from build123d import *

# Parameters (mm, degrees)
F1_DEPTH  = 1
F0_W      = 50
F0_H      = 23.8363201171
F0_W_2    = 35
F2_DEPTH  = 4
F3_W      = 50
F3_H      = 5
F3_H_2    = 13.8363201171
F4_DEPTH  = 20
F6_DEPTH  = 50
F7_W      = 4
F7_H      = 10
F7_H_2    = 6.0470494551
F8_DEPTH  = 12
F9_START  = -7
F7_W_2    = 1.75
F9_DEPTH  = 5
F10_W     = 23
F10_H     = 5
F11_DEPTH = 45


with BuildPart() as f1:
    # F0 (on Top) → F1 (new body)
    with BuildSketch(Plane.XY):
        Polygon((-50, 46.1636798829), (-50, 23.8363201171), (-25, 23.8363201171), (25, 23.8363201171), (50, 23.8363201171), (50, 46.1636798829), (15, 46.1636798829), (15, 70), (-15, 70), (-15, 46.1636798829), align=None)
    extrude(amount=F1_DEPTH)

    # F0 (on Top) → F2 (join)
    with BuildSketch(Plane.XY):
        with Locations((0, 11.9181600586)):
            Rectangle(F0_W, F0_H)
        with Locations((32.5, 58.0818399414)):
            Rectangle(F0_W_2, F0_H)
        with Locations((-32.5, 58.0818399414)):
            Rectangle(F0_W_2, F0_H)
    extrude(amount=F2_DEPTH)

    # F3 (on face) → F4 (join)
    with BuildSketch(Plane.XY.offset(4)):
        with Locations((0, 21.3363201171)):
            Rectangle(F3_W, F3_H)
        with Locations((0, 11.9181600586)):
            Rectangle(F3_W, F3_H_2)
        with Locations((0, 2.5)):
            Rectangle(F3_W, F3_H)
    extrude(amount=F4_DEPTH)

    # F5 (on face) → F6 (cut)
    with BuildSketch(Plane.YZ.offset(25)):
        Polygon((0, 24), (0, 4), (5, 24), align=None)
        Polygon((22.7283012867, 19.5679246783), (18.8363201171, 4), (23.8363201171, 4), (23.8363201171, 24), align=None)
        Polygon((23.8363201171, 24), (5, 24), (22.7283012867, 19.5679246783), align=None)
    extrude(amount=-F6_DEPTH, mode=Mode.SUBTRACT)

    # F7 (on face) → F8 (cut)
    with BuildSketch(Plane(origin=(0, 16.7871248161, -4.196781204), x_dir=(-1, 0, 0), z_dir=(0, 0.9701425001, -0.242535625))):
        with Locations((0, 19.4960981287)):
            Rectangle(F7_W, F7_H)
        with Locations((0, 11.4725734011)):
            Rectangle(F7_W, F7_H_2)
    extrude(amount=-F8_DEPTH, mode=Mode.SUBTRACT)

    # F7 (on face) → F9 (cut)
    with BuildSketch(Plane(origin=(0, 16.7871248161, -4.196781204), x_dir=(-1, 0, 0), z_dir=(0, 0.9701425001, -0.242535625)).offset(F9_START)):
        with Locations((2.875, 19.4960981287)):
            Rectangle(F7_W_2, F7_H)
        with Locations((-2.875, 19.4960981287)):
            Rectangle(F7_W_2, F7_H)
    extrude(amount=-F9_DEPTH, mode=Mode.SUBTRACT)

    # F10 (on face) → F11 (join)
    with BuildSketch(Plane(origin=(0, 5.9411764706, 23.7647058824), x_dir=(1, 0, 0), z_dir=(0, 0.242535625, 0.9701425001))):
        Polygon((40, 17.3037721918), (25, 17.3037721918), (25, 12.3037721918), (35, 12.3037721918), (35, -7.6962278082), (40, -7.6962278082), align=None)
        with Locations((13.5, 14.8037721918)):
            Rectangle(F10_W, F10_H)
        with Locations((-13.5, 14.8037721918)):
            Rectangle(F10_W, F10_H)
        Polygon((-25, 17.3037721918), (-40, 17.3037721918), (-40, -7.6962278082), (-35, -7.6962278082), (-35, 12.3037721918), (-25, 12.3037721918), align=None)
    extrude(amount=F11_DEPTH)


solid = f1.part
Could you check a few things on this model? Use its own coordinates, in mm. A direction names the side the tool comes from. Give positions to 0.01 mm unless a question says otherwise; leave off trailing zeros. Order: outer loops, then holes, each group sorted by start corner. A loop starts at its lowest first (then second) coordinate and runs counter-clockwise, first axis right, second up.
1. We'd pull the mould along Y, two halves only. Please class faces 4 (the flat face through (37.465, 3.855, 47.154)), 5 (the flat face through (-1, 43, 0)), 6 (the flat face through (0.05, 9.6, 16.53)): pulls with the +Y half, pulls with the -Y half, needs draft (parallel to the pull), parting line crosses it, or undercut.
2. Suppose I cut it at A-A (x = -32). List the corners of the cut face in (y, z) for me, plus the area to 3 significant figures.
3. For faces 1 (the flat face through (-33, 46.164, 2)), 2 (the flat face through (-2.86, 14.74, 16.48)), 3 (the flat face through (0, 21, 4)), which set-ups out of +Z, -Z, +X, -X, +Y, -Y let a thin tool reach every point of the face, with its end or its side?
4. Will these pins go through, and if not, where does the flat tip stop? P1, Ø0.8, axis at x = 40, z = 0.5, coming from the -Y side; P2, Ø0.9, axis at x = -33.5, z = 3, coming from the -Y side; P3, Ø13, axis at y = 18.5, z = 26.5, coming from the -X side.
5. Suppose I cut it at C-C (z = 38). List the corners of the cut face in (x, y) for me.
6. Suppose I cut it at D-D (y = 49.5). List the corners of the cut face in (x, z) for me, plus the area to 3 significant figures.
7. I need wall thicknesses on L1, parallel to X at y = 27.5, z = 41.5; L2, parallel to X at y = 20, z = 36; L3, parallel to Z at x = -33.5, y = 61. Which ranges of each line are inside material? Lowest first, please.
8. Suppose I cut it at B-B (x = 17). List the corners of the cut face in (y, z) for me, plus the area to 3 significant figures.
Solved:
1. face 4: pulls with the -Y half
1. face 5: needs draft
1. face 6: undercut
2. outline: (17.88, 20.78) - (22.73, 19.57) - (33.64, 63.22) - (28.79, 64.44) - close; (23.84, 0) - (70, 0) - (70, 4) - (46.16, 4) - (46.16, 1) - (23.84, 1) - close
2. area: 343 mm2
3. face 1: +Z, +X, -X
3. face 2: +Z
3. face 3: +X, -X, +Y
4. P1: stops at y = 23.84
4. P2: stops at y = 46.16
4. P3: stops at x = -40
5. outline: (-40, 1.57) - (-35, 1.57) - (-35, 22.18) - (-2, 22.18) - (-2, 27.34) - (-40, 27.34) - close; (2, 22.18) - (35, 22.18) - (35, 1.57) - (40, 1.57) - (40, 27.34) - (2, 27.34) - close
6. outline: (-50, 0) - (50, 0) - (50, 4) - (15, 4) - (15, 1) - (-15, 1) - (-15, 4) - (-50, 4) - close
6. area: 310 mm2
7. L1: x = -40 to -2, 2 to 40
7. L2: x = -40 to -35, 35 to 40
7. L3: z = 0 to 4
8. outline: (0, 0) - (70, 0) - (70, 4) - (46.16, 4) - (46.16, 1) - (23.84, 1) - (23.84, 4) - (18.84, 4) - (33.64, 63.22) - (28.79, 64.44) - (17.88, 20.78) - (5, 24) - (0, 4) - close
8. area: 773 mm2
